from build123d import *

# Parameters (mm, degrees)
EXTRUSION1_DEPTH = 17
ESQUISSE2_R      = 1.5
EXTRUSION2_DEPTH = 15


with BuildPart() as part:
    # Esquisse1 → Extrusion1 (new body)
    with BuildSketch(Plane.XY):
        Polygon((-21.976949538, -4.544631579), (-21.976949538, -19.544631579), (-6.976949538, -19.544631579), (-6.976949538, -18.044631579), (-20.476949538, -18.044631579), (-20.476949538, -4.544631579), align=None)
    extrude(amount=EXTRUSION1_DEPTH)

    # Esquisse2 → Extrusion2 (cut)
    with BuildSketch(Plane(origin=(0, -18.044631579, 0), x_dir=(1, 0, 0), z_dir=(0, 1, 0))):
        with Locations(Location((-16.476949538, -13.5, 0), (0, 0, 180))):
            Circle(ESQUISSE2_R)
        with Locations(Location((-16.476949538, -3.5, 0), (0, 0, 180))):
            Circle(ESQUISSE2_R)
    extrude(amount=-EXTRUSION2_DEPTH, mode=Mode.SUBTRACT)


solid = part.part
Work out the finished part from the listing and answer in its coordinate system (mm). A direction names the side the tool comes from. Give positions to 0.01 mm unless a question says otherwise; leave off trailing zeros. Write each loop counter-clockwise with the first axis right and the second up, starting at its lowest first coordinate (ties: lowest second). Pieces come first, ordered by that corner, then holes. Notation, with made-up numbers: M 81.5,81 L 100.5,81 A26 ccw 100.5,102 Z; hole C 67,70.5 d6. An arc over 180 degrees is marked long. Answer as CSV lines item,"result".
Q1. A cutting plane is placed at B-B on x = -15.25. Write down the section's boundary in (y, z).
A:
outline,"M -19.54,0 L -18.04,0 L -18.04,2.64 L -19.54,2.64 Z; M -19.54,4.36 L -18.04,4.36 L -18.04,12.64 L -19.54,12.64 Z; M -19.54,14.36 L -18.04,14.36 L -18.04,17 L -19.54,17 Z"
Q2. A cutting plane is placed at C-C on z = 9.5. Write down the section's boundary in (x, y).
A:
outline,"M -21.98,-19.54 L -6.98,-19.54 L -6.98,-18.04 L -20.48,-18.04 L -20.48,-4.54 L -21.98,-4.54 Z"
Q3. Find the intervals of material crossed by probe 1 along Y at (x, z) = (-16.5, 11.75); probe 2 along X at (y, z) = (-11.75, 11.25), in increasing order. Write a range as [from, to].
A:
probe 1,"y = [-19.54, -18.04]"
probe 2,"x = [-21.98, -20.48]"
Q4. The mould has two halves that part along Z. Classify faces 1 (the cylindrical face through (-17.908, -18.784, 3.951)), 2 (the flat face through (-15, -19.545, 8)), 3 (the flat face through (-21, -15, 0)): +Z half, -Z half, draft (parallel to the pull), parting line (faces both ways), or undercut.
A:
face 1,"undercut"
face 2,"draft"
face 3,"-Z half"
Q5. A cutting plane is placed at A-A on z = 13.5. Write down the section's boundary in (x, y), plus the area to 4 significant figures.
A:
outline,"M -21.98,-19.54 L -17.98,-19.54 L -17.98,-18.04 L -20.48,-18.04 L -20.48,-4.54 L -21.98,-4.54 Z; M -14.98,-19.54 L -6.98,-19.54 L -6.98,-18.04 L -14.98,-18.04 Z"
area,"38.25 mm²"
Q6. A cutting plane is placed at D-D on y = -13. Write down the section's boundary in (x, z).
A:
outline,"M -21.98,0 L -20.48,0 L -20.48,17 L -21.98,17 Z"
Q7. A tool of negligible diameter and unlimited length cuts with its end or side. For faces 4 (the cylindrical face through (-17.908, -18.784, 13.951)), 5 (the flat face through (-14, -18.045, 8)), from which of +Z, -Z, +X, -X, +Y, -Y can it reach the whole face along a straight path? Write none if from no direction.
A:
face 4,"+Y, -Y"
face 5,"+Z, -Z, +X, +Y"
Q8. Given P1, Ø2, axis at x = -16, z = 2.5, coming from the +Y side; P2, Ø8, axis at x = -14.5, y = -11.5, coming from the +Z side, each flat-ended and moving along its own axis, determine where each tip first touches the part or whether it passes through.
A:
P1,"stops at y = -18.04"
P2,"passes through"
